Read the model definition and answer for the solid it produces. Units are mm, in the model's axes. Face numbers are marked on the shaded views. A direction names the side the tool comes from. Round coordinates to 2 decimals unless told otherwise and drop trailing zeros. Write each loop counter-clockwise with the first axis right and the second up, starting at its lowest first coordinate (ties: lowest second). Pieces come first, ordered by that corner, then holes. Notation, with made-up numbers: (27.25, 32.25) -> (54.25, 32.25) arc R18 cw to (54.25, 53.25) -> close; hole circle Ø11 at (-39.75, 53.25). An arc over 180 degrees is marked (long way). Return JSON: item names as keys, results as strings.
from build123d import *

# Parameters (mm, degrees)
SKETCH_1_R          = 1.5
EXTRUDE_1_DEPTH     = 2
SKETCH_2_W          = 2
SKETCH_2_H          = 20
EXTRUDE_2_DEPTH     = 14
SKETCH_4_R          = 3.75
CUT_EXTRUDE_1_DEPTH = 10


with BuildPart() as part:
    # 草图1 → 凸台-拉伸1 (new body)
    with BuildSketch(Plane(origin=(0, 0, 0), x_dir=(1, 0, 0), z_dir=(0, 1, 0))):
        Polygon((-3, 0), (-3, -10), (15, -10), (15, 10), (-3, 10), align=None)
        with Locations((3, 0)):
            Circle(SKETCH_1_R, mode=Mode.SUBTRACT)
        with Locations((11, 5)):
            Circle(SKETCH_1_R, mode=Mode.SUBTRACT)
        with Locations((11, -5)):
            Circle(SKETCH_1_R, mode=Mode.SUBTRACT)
    extrude(amount=EXTRUDE_1_DEPTH)

    # 草图2 → 凸台-拉伸2 (add)
    with BuildSketch(Plane(origin=(0, 2, 0), x_dir=(1, 0, 0), z_dir=(0, 1, 0))):
        with Locations((-2, 0)):
            Rectangle(SKETCH_2_W, SKETCH_2_H)
    extrude(amount=EXTRUDE_2_DEPTH)

    # 草图4 → 切除-拉伸1 (cut)
    with BuildSketch(Plane(origin=(-1, 0, 0), x_dir=(0, 0, -1), z_dir=(1, 0, 0))):
        with Locations((0, 9)):
            Circle(SKETCH_4_R)
    extrude(amount=-CUT_EXTRUDE_1_DEPTH, mode=Mode.SUBTRACT)

    # 草图7 → 切除-旋转1 (revolve, cut)
    with BuildSketch(Plane(origin=(0, 2, 0), x_dir=(1, 0, 0), z_dir=(0, 1, 0))):
        Polygon((7, 0), (15, 0), (15, 1.5), align=None)
    revolve(axis=Axis((7, 2, 0), (1, 0, 0)), mode=Mode.SUBTRACT)


solid = part.part
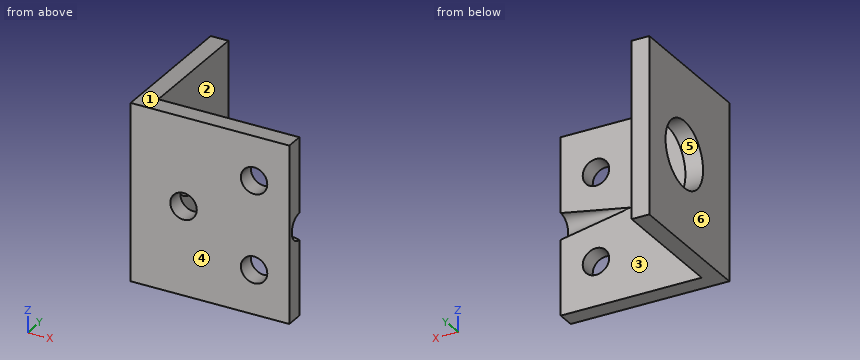
Item 1: Flat-ended cylindrical pins translate along their axes: pin 1 (2 mm diameter, centred on x = 2.5, z = 7, fed in from -Y); pin 2 (3 mm diameter, centred on x = 12.5, z = -4.5, fed in from +Y); pin 3 (3 mm diameter, centred on y = 10, z = 7, fed in from +X). Find the tip coordinate at first contact, or state that the pin passes through.
Worked answers:
{"pin 1": "stops at y = 0", "pin 2": "stops at y = 2", "pin 3": "stops at x = -1"}
Item 2: Section D-D (z = 0) is taken. Give the vertices of the cut face in (x, y).
Worked answers:
{"outline": "(-3, 0) -> (1.5, 0) -> (1.5, 2) -> (-1, 2) -> (-1, 5.25) -> (-3, 5.25) -> close; (-3, 12.75) -> (-1, 12.75) -> (-1, 16) -> (-3, 16) -> close; (4.5, 0) -> (15, 0) -> (15, 0.5) -> (7, 2) -> (4.5, 2) -> close"}
Item 3: For a pull along Y with two mould halves and no side action, classify the marked faces 3, 4, 5 and 6 as released by +Y, released by -Y, zero draft, split by the parting line, or undercut.
Worked answers:
{"face 3": "released by +Y", "face 4": "released by -Y", "face 5": "undercut", "face 6": "zero draft"}
Item 4: Section A-A (z = -5) is taken. Give the vertices of the cut face in (x, y), then the cut area to 3 significant figures.
Worked answers:
{"outline": "(-3, 0) -> (9.5, 0) -> (9.5, 2) -> (-1, 2) -> (-1, 16) -> (-3, 16) -> close; (12.5, 0) -> (15, 0) -> (15, 2) -> (12.5, 2) -> close", "area": "58.0 mm2"}
Item 5: Straight lines are drawn through the part: L1, parallel to Z at x = 11, y = 1.05; L2, parallel to Z at x = 3, y = 0.5; L3, parallel to X at y = 1.2, z = 5. For each, find the intervals that lie inside material, in ascending order. Write a range as [from, to].
Worked answers:
{"L1": "z = [-10, -6.5], [-3.5, 3.5], [6.5, 10]", "L2": "z = [-10, -1.5], [1.5, 10]", "L3": "x = [-3, 9.5], [12.5, 15]"}
Item 6: Section C-C (y = 11.25) is taken. Give the vertices of the cut face in (x, z), then the cut area to 3 significant figures.
Worked answers:
{"outline": "(-3, -10) -> (-1, -10) -> (-1, -3) -> (-3, -3) -> close; (-3, 3) -> (-1, 3) -> (-1, 10) -> (-3, 10) -> close", "area": "28.0 mm2"}
Item 7: Section B-B (x = 3) is taken. Give the vertices of the cut face in (y, z).
Worked answers:
{"outline": "(0, -10) -> (2, -10) -> (2, -1.5) -> (0, -1.5) -> close; (0, 1.5) -> (2, 1.5) -> (2, 10) -> (0, 10) -> close"}
Item 8: A tool of negligible diameter and unlimited length cuts with its end or side. For the marked faces 1 and 2, from which of +Z, -Z, +X, -X, +Y, -Y can it reach the whole face along a straight path? Write none if from no direction.
Worked answers:
{"face 1": "+Z, +X, -X, +Y, -Y", "face 2": "+Z, -Z, +X, +Y"}
